from build123d import *

# Parameters (mm, degrees)
SKETCH_1_W          = 170
SKETCH_1_H          = 70
EXTRUDE_1_DEPTH     = 2
SKETCH_2_R          = 5.5
CUT_EXTRUDE_1_DEPTH = 92.945636112
CUT_EXTRUDE_2_DEPTH = 92.945636112


with BuildPart() as part:
    # 草圖1 → 填料-伸長1 (new body)
    with BuildSketch(Plane.XY):
        Rectangle(SKETCH_1_W, SKETCH_1_H)
    extrude(amount=EXTRUDE_1_DEPTH)

    # 草圖2 → 除料-伸長1 (cut, through all)
    with BuildSketch(Plane.XY.offset(2)):
        Circle(SKETCH_2_R)
        with BuildLine():
            Line((43.5, -22.5), (43.5, 22.5))
            ThreePointArc((43.5, 22.5), (45, 24), (46.5, 22.5))
            Line((46.5, 22.5), (46.5, -22.5))
            ThreePointArc((46.5, -22.5), (45, -24), (43.5, -22.5))
        make_face()
        with BuildLine():
            Line((-46.5, -22.5), (-46.5, 22.5))
            ThreePointArc((-46.5, 22.5), (-45, 24), (-43.5, 22.5))
            Line((-43.5, 22.5), (-43.5, -22.5))
            ThreePointArc((-43.5, -22.5), (-45, -24), (-46.5, -22.5))
        make_face()
        with BuildLine():
            Line((21.5, 28.5), (8.5, 28.5))
            ThreePointArc((8.5, 28.5), (7, 30), (8.5, 31.5))
            Line((8.5, 31.5), (21.5, 31.5))
            ThreePointArc((21.5, 31.5), (23, 30), (21.5, 28.5))
        make_face()
        with BuildLine():
            Line((-82.5, -22.5), (-82.5, 22.5))
            ThreePointArc((-82.5, 22.5), (-81, 24), (-79.5, 22.5))
            Line((-79.5, 22.5), (-79.5, -22.5))
            ThreePointArc((-79.5, -22.5), (-81, -24), (-82.5, -22.5))
        make_face()
        with BuildLine():
            Line((79.5, -22.5), (79.5, 22.5))
            ThreePointArc((79.5, 22.5), (81, 24), (82.5, 22.5))
            Line((82.5, 22.5), (82.5, -22.5))
            ThreePointArc((82.5, -22.5), (81, -24), (79.5, -22.5))
        make_face()
        with BuildLine():
            Line((21.5, 21), (8.5, 21))
            ThreePointArc((8.5, 21), (7, 22.5), (8.5, 24))
            Line((8.5, 24), (21.5, 24))
            ThreePointArc((21.5, 24), (23, 22.5), (21.5, 21))
        make_face()
        with BuildLine():
            Line((-21.5, 28.5), (-8.5, 28.5))
            ThreePointArc((-8.5, 28.5), (-7, 30), (-8.5, 31.5))
            Line((-8.5, 31.5), (-21.5, 31.5))
            ThreePointArc((-21.5, 31.5), (-23, 30), (-21.5, 28.5))
        make_face()
        with BuildLine():
            Line((-21.5, 21), (-8.5, 21))
            ThreePointArc((-8.5, 21), (-7, 22.5), (-8.5, 24))
            Line((-8.5, 24), (-21.5, 24))
            ThreePointArc((-21.5, 24), (-23, 22.5), (-21.5, 21))
        make_face()
        with BuildLine():
            Line((21.5, -28.5), (8.5, -28.5))
            ThreePointArc((8.5, -28.5), (7, -30), (8.5, -31.5))
            Line((8.5, -31.5), (21.5, -31.5))
            ThreePointArc((21.5, -31.5), (23, -30), (21.5, -28.5))
        make_face()
        with BuildLine():
            Line((21.5, -21), (8.5, -21))
            ThreePointArc((8.5, -21), (7, -22.5), (8.5, -24))
            Line((8.5, -24), (21.5, -24))
            ThreePointArc((21.5, -24), (23, -22.5), (21.5, -21))
        make_face()
        with BuildLine():
            Line((-21.5, -28.5), (-8.5, -28.5))
            ThreePointArc((-8.5, -28.5), (-7, -30), (-8.5, -31.5))
            Line((-8.5, -31.5), (-21.5, -31.5))
            ThreePointArc((-21.5, -31.5), (-23, -30), (-21.5, -28.5))
        make_face()
        with BuildLine():
            Line((-21.5, -21), (-8.5, -21))
            ThreePointArc((-8.5, -21), (-7, -22.5), (-8.5, -24))
            Line((-8.5, -24), (-21.5, -24))
            ThreePointArc((-21.5, -24), (-23, -22.5), (-21.5, -21))
        make_face()
    extrude(amount=-CUT_EXTRUDE_1_DEPTH, mode=Mode.SUBTRACT)

    # 草圖4 → 除料-伸長2 (cut, through all)
    with BuildSketch(Plane.XY.offset(2)):
        with BuildLine():
            Line((85, 35), (33, 35))
            ThreePointArc((33, 35), (34.414213562, 34.414213562), (35, 33))
            Line((35, 33), (35, 29))
            ThreePointArc((35, 29), (35.585786438, 27.585786438), (37, 27))
            Line((37, 27), (83, 27))
            ThreePointArc((83, 27), (84.414213562, 26.414213562), (85, 25))
            Line((85, 25), (85, 35))
        make_face()
        with BuildLine():
            Line((35, -33), (35, -29))
            ThreePointArc((35, -29), (35.585786438, -27.585786438), (37, -27))
            Line((37, -27), (83, -27))
            ThreePointArc((83, -27), (84.414213562, -26.414213562), (85, -25))
            Line((85, -25), (85, -35))
            Line((85, -35), (33, -35))
            ThreePointArc((33, -35), (34.414213562, -34.414213562), (35, -33))
        make_face()
        with BuildLine():
            Line((-85, -35), (-33, -35))
            ThreePointArc((-33, -35), (-34.414213562, -34.414213562), (-35, -33))
            Line((-35, -33), (-35, -29))
            ThreePointArc((-35, -29), (-35.585786438, -27.585786438), (-37, -27))
            Line((-37, -27), (-83, -27))
            ThreePointArc((-83, -27), (-84.414213562, -26.414213562), (-85, -25))
            Line((-85, -25), (-85, -35))
        make_face()
        with BuildLine():
            Line((-35, 33), (-35, 29))
            ThreePointArc((-35, 29), (-35.585786438, 27.585786438), (-37, 27))
            Line((-37, 27), (-83, 27))
            ThreePointArc((-83, 27), (-84.414213562, 26.414213562), (-85, 25))
            Line((-85, 25), (-85, 35))
            Line((-85, 35), (-33, 35))
            ThreePointArc((-33, 35), (-34.414213562, 34.414213562), (-35, 33))
        make_face()
    extrude(amount=-CUT_EXTRUDE_2_DEPTH, mode=Mode.SUBTRACT)


solid = part.part
Input: part model. Units: mm. Frame: model coordinates. Coordinates: 2 decimals unless noted, no trailing zeros. Loops run counter-clockwise (first coordinate to the right, second up) from the corner with the lowest first, then second, coordinate; pieces in that order, holes last. Notation, with made-up numbers: (-5.5, 19) -> (2.5, 19) arc R12 ccw to (2.5, 24) -> close; hole circle Ø4 at (-22, -8). An arc over 180 degrees is marked (long way). Write each question's results on one line, items separated by ' | '. Start each with the question number.
Q1. Section B-B, the plane y = 14.5. Return the cut outline in (x, z).
Q2. Section A-A, the plane x = -81. Return the cut outline in (y, z), plus the area to 3 significant figures.
Q3. Ray query, line 1 (Y direction, x = -14, z = 1.05); line 2 (X direction, y = -8, z = 1.8); line 3 (Y direction, x = 0, z = 1.25). Return the intervals inside material, ascending. Write a range as from..to.
Q4. Pull-direction query (Y, two-part tool) for faces 1 (the cylindrical face through (-1.19, -5.37, 1.01)), 2 (the flat face through (-1, 8, 0)); classes: released by +Y, released by -Y, zero draft, split by the parting line, or undercut.
Q5. Pin query (flat end, axial travel): pin 1 (0.6 mm diameter, centred on x = 62, z = 0.5, fed in from +Y); pin 2 (1 mm diameter, centred on y = 31.5, z = 0.5, fed in from +X). Return the tip coordinate at first contact, or that it passes through.
Q6. Section C-C, the plane y = 3. Return the cut outline in (x, z).
Q7. Section D-D, the plane z = 0.5. State how many separate pieces and enclosed holes the cut face has, plus the area to 3 significant figures.
Found:
1) outline: (-85, 0) -> (-82.5, 0) -> (-82.5, 2) -> (-85, 2) -> close; (-79.5, 0) -> (-46.5, 0) -> (-46.5, 2) -> (-79.5, 2) -> close; (-43.5, 0) -> (43.5, 0) -> (43.5, 2) -> (-43.5, 2) -> close; (46.5, 0) -> (79.5, 0) -> (79.5, 2) -> (46.5, 2) -> close; (82.5, 0) -> (85, 0) -> (85, 2) -> (82.5, 2) -> close
2) outline: (-27, 0) -> (-24, 0) -> (-24, 2) -> (-27, 2) -> close; (24, 0) -> (27, 0) -> (27, 2) -> (24, 2) -> close | area: 12.0 mm2
3) line 1: -35..-31.5, -28.5..-24, -21..21, 24..28.5, 31.5..35 | line 2: -85..-82.5, -79.5..-46.5, -43.5..43.5, 46.5..79.5, 82.5..85 | line 3: -35..-5.5, 5.5..35
4) face 1: undercut | face 2: zero draft
5) pin 1: y = 27 | pin 2: x = 35
6) outline: (-85, 0) -> (-82.5, 0) -> (-82.5, 2) -> (-85, 2) -> close; (-79.5, 0) -> (-46.5, 0) -> (-46.5, 2) -> (-79.5, 2) -> close; (-43.5, 0) -> (-4.61, 0) -> (-4.61, 2) -> (-43.5, 2) -> close; (4.61, 0) -> (43.5, 0) -> (43.5, 2) -> (4.61, 2) -> close; (46.5, 0) -> (79.5, 0) -> (79.5, 2) -> (46.5, 2) -> close; (82.5, 0) -> (85, 0) -> (85, 2) -> (82.5, 2) -> close
7) separate pieces: 1 | enclosed holes: 13 | area: 9,260 mm2
